The listing builds one solid part. Answer for the finished solid, in the listing's coordinates (mm). Face numbers are marked on the shaded views. Coordinates: 2 decimals unless noted, no trailing zeros. Order: outer loops, then holes, each group sorted by start corner. A loop starts at its lowest first (then second) coordinate and runs counter-clockwise, first axis right, second up. Notation, with made-up numbers: M 46.25,74.25 L 82.25,74.25 A8 cw 82.25,79.25 Z; hole C -21,-28.75 d1. An arc over 180 degrees is marked long. One line per item, written item: value. Start each with the question number.
Q1. Each of these flat-tipped pins is pushed along its axis until it touches: pin 1 Ø2 at (y, z) = (-5.5, -104) entering from -X; pin 2 Ø2 at (x, z) = (66.5, -6.5) entering from -Y; pin 3 Ø4 at (y, z) = (-22.5, -83) entering from -X. Where does it stop, or does it pass through?
Q2. Straight lines are drawn through the part: line 1 along X through (y, z) = (-5, -84); line 2 along Y through (x, z) = (62.5, -21.5); line 3 along Y through (x, z) = (81, -77). For each, find the intervals that lie inside material, in ascending order. Write a range as [from, to].
Q3. The part is cut by section A-A on y = -2. Give the vertices of the cut face in (x, z), then the cut area to 3 significant figures.
Q4. Determine the mould class of the marked faces 1 and 2 for opening direction Z: pulls with the +Z half, pulls with the -Z half, needs draft (parallel to the pull), parting line crosses it, or undercut.
```python
from build123d import *

# Parameters (mm, degrees)
SKETCH1_W                       = 24.199471414
SKETCH1_H                       = 2
BOSS_EXTRUDE1_DEPTH             = 35
BOSS_EXTRUDE1_DIRECTION_2_REACH = 26.277


with BuildPart() as part:
    # Sketch6 → Revolve3 (revolve)
    with BuildSketch(Plane.XY.offset(-46.235660898)):
        with BuildLine():
            Line((16.206828031, 19.733449427), (16.206828031, 24.27673627))
            add(Edge.make_bspline(
                [(100.543718281, 0), (66.637702737, 19.683925925), (36.295673337, 23.877083975), (16.206828031, 24.27673627)],
                knots=[0, 0, 0, 0, 1, 1, 1, 1], degree=3))
            add(Edge.make_bspline(
                [(16.206828031, 19.733449427), (44.550281864, 20.046720972), (71.658331759, 8.477286849), (100.543718281, 0)],
                knots=[0, 0, 0, 0, 1, 1, 1, 1], degree=3))
        make_face()
    revolve(axis=Axis((16.206828031, 19.733449427, -46.235660898), (0, 1, 0)))

    # Sketch1 → Boss-Extrude1 (add)
    with BuildSketch(Plane(origin=(0, 0, 0), x_dir=(1, 0, 0), z_dir=(0, 1, 0))):
        with Locations((19.440545507, 104.374561644)):
            Rectangle(SKETCH1_W, SKETCH1_H)
        Polygon((68.633841253, 77.067834217), (57.432693736, 91.113628939), (55.869030771, 89.866649335), (69.659558116, 72.573875009), align=None)
        Polygon((72.129937387, 19.465930814), (77.514826367, 43.058670955), (75.564970543, 43.503712823), (70.180081563, 19.910972681), align=None)
        Polygon((30.661981859, -13.103705945), (52.464952222, -2.603948803), (51.597184744, -0.802011068), (29.79421438, -11.301768209), align=None)
        Polygon((-20.656832908, -0.989589169), (1.146137456, -11.48934631), (2.013904934, -9.687408574), (-19.78906543, 0.812348567), align=None)
        Polygon((-43.18239268, 46.686104127), (-37.7975037, 23.093363986), (-35.847647875, 23.538405854), (-41.232536856, 47.131145995), align=None)
        Polygon((-19.952491512, 94.022604484), (-35.040615149, 75.102695874), (-33.476952184, 73.85571627), (-18.388828547, 92.77562488), align=None)
    extrude(amount=-BOSS_EXTRUDE1_DEPTH)

    # Sketch1 → Boss-Extrude1 direction 2 (add, up to next)
    with BuildSketch(Plane(origin=(0, 0, 0), x_dir=(1, 0, 0), z_dir=(0, 1, 0)), mode=Mode.PRIVATE) as boss_extrude1_direction_2_sk1:
        with Locations((19.440545507, 104.374561644)):
            Rectangle(SKETCH1_W, SKETCH1_H)
    boss_extrude1_direction_2_tool1 = extrude(boss_extrude1_direction_2_sk1.sketch, amount=BOSS_EXTRUDE1_DIRECTION_2_REACH, mode=Mode.PRIVATE) - part.part
    add(boss_extrude1_direction_2_tool1.solids().sort_by_distance((19.440546, 0, -104.374562))[0])
    # Sketch1 → Boss-Extrude1 direction 2 (add, up to next)
    with BuildSketch(Plane(origin=(0, 0, 0), x_dir=(1, 0, 0), z_dir=(0, 1, 0)), mode=Mode.PRIVATE) as boss_extrude1_direction_2_sk2:
        Polygon((68.633841253, 77.067834217), (57.432693736, 91.113628939), (55.869030771, 89.866649335), (69.659558116, 72.573875009), align=None)
    boss_extrude1_direction_2_tool2 = extrude(boss_extrude1_direction_2_sk2.sketch, amount=BOSS_EXTRUDE1_DIRECTION_2_REACH, mode=Mode.PRIVATE) - part.part
    add(boss_extrude1_direction_2_tool2.solids().sort_by_distance((62.894136, 0, -82.605929))[0])
    # Sketch1 → Boss-Extrude1 direction 2 (add, up to next)
    with BuildSketch(Plane(origin=(0, 0, 0), x_dir=(1, 0, 0), z_dir=(0, 1, 0)), mode=Mode.PRIVATE) as boss_extrude1_direction_2_sk3:
        Polygon((72.129937387, 19.465930814), (77.514826367, 43.058670955), (75.564970543, 43.503712823), (70.180081563, 19.910972681), align=None)
    boss_extrude1_direction_2_tool3 = extrude(boss_extrude1_direction_2_sk3.sketch, amount=BOSS_EXTRUDE1_DIRECTION_2_REACH, mode=Mode.PRIVATE) - part.part
    add(boss_extrude1_direction_2_tool3.solids().sort_by_distance((73.847454, 0, -31.484822))[0])
    # Sketch1 → Boss-Extrude1 direction 2 (add, up to next)
    with BuildSketch(Plane(origin=(0, 0, 0), x_dir=(1, 0, 0), z_dir=(0, 1, 0)), mode=Mode.PRIVATE) as boss_extrude1_direction_2_sk4:
        Polygon((30.661981859, -13.103705945), (52.464952222, -2.603948803), (51.597184744, -0.802011068), (29.79421438, -11.301768209), align=None)
    boss_extrude1_direction_2_tool4 = extrude(boss_extrude1_direction_2_sk4.sketch, amount=BOSS_EXTRUDE1_DIRECTION_2_REACH, mode=Mode.PRIVATE) - part.part
    add(boss_extrude1_direction_2_tool4.solids().sort_by_distance((41.129583, 0, 6.952859))[0])
    # Sketch1 → Boss-Extrude1 direction 2 (add, up to next)
    with BuildSketch(Plane(origin=(0, 0, 0), x_dir=(1, 0, 0), z_dir=(0, 1, 0)), mode=Mode.PRIVATE) as boss_extrude1_direction_2_sk5:
        Polygon((-20.656832908, -0.989589169), (1.146137456, -11.48934631), (2.013904934, -9.687408574), (-19.78906543, 0.812348567), align=None)
    boss_extrude1_direction_2_tool5 = extrude(boss_extrude1_direction_2_sk5.sketch, amount=BOSS_EXTRUDE1_DIRECTION_2_REACH, mode=Mode.PRIVATE) - part.part
    add(boss_extrude1_direction_2_tool5.solids().sort_by_distance((-9.321464, 0, 5.338499))[0])
    # Sketch1 → Boss-Extrude1 direction 2 (add, up to next)
    with BuildSketch(Plane(origin=(0, 0, 0), x_dir=(1, 0, 0), z_dir=(0, 1, 0)), mode=Mode.PRIVATE) as boss_extrude1_direction_2_sk6:
        Polygon((-43.18239268, 46.686104127), (-37.7975037, 23.093363986), (-35.847647875, 23.538405854), (-41.232536856, 47.131145995), align=None)
    boss_extrude1_direction_2_tool6 = extrude(boss_extrude1_direction_2_sk6.sketch, amount=BOSS_EXTRUDE1_DIRECTION_2_REACH, mode=Mode.PRIVATE) - part.part
    add(boss_extrude1_direction_2_tool6.solids().sort_by_distance((-39.51502, 0, -35.112255))[0])
    # Sketch1 → Boss-Extrude1 direction 2 (add, up to next)
    with BuildSketch(Plane(origin=(0, 0, 0), x_dir=(1, 0, 0), z_dir=(0, 1, 0)), mode=Mode.PRIVATE) as boss_extrude1_direction_2_sk7:
        Polygon((-19.952491512, 94.022604484), (-35.040615149, 75.102695874), (-33.476952184, 73.85571627), (-18.388828547, 92.77562488), align=None)
    boss_extrude1_direction_2_tool7 = extrude(boss_extrude1_direction_2_sk7.sketch, amount=BOSS_EXTRUDE1_DIRECTION_2_REACH, mode=Mode.PRIVATE) - part.part
    add(boss_extrude1_direction_2_tool7.solids().sort_by_distance((-26.714722, 0, -83.93916))[0])


solid = part.part
```
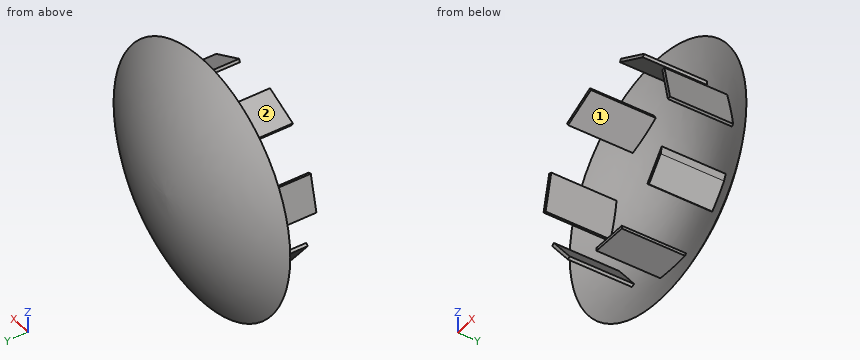
Output:
1. pin 1: stops at x = 7.34
1. pin 2: stops at y = 6.01
1. pin 3: stops at x = -30.34
2. line 1: x = [-27.95, -25.39], [60.55, 63.11]
2. line 2: y = [10.03, 14.74]
2. line 3: y = [3.88, 6.72]
3. outline: M -43.18,-46.69 L -41.23,-47.13 L -35.85,-23.54 L -37.8,-23.09 Z; M -35.04,-75.1 L -19.95,-94.02 L -18.39,-92.78 L -33.48,-73.86 Z; M -20.66,0.99 L -19.79,-0.81 L 2.01,9.69 L 1.15,11.49 Z; M 7.34,-105.37 L 31.54,-105.37 L 31.54,-103.37 L 7.34,-103.37 Z; M 29.79,11.3 L 51.6,0.8 L 52.46,2.6 L 30.66,13.1 Z; M 55.87,-89.87 L 57.43,-91.11 L 68.63,-77.07 L 69.66,-72.57 Z; M 70.18,-19.91 L 75.56,-43.5 L 77.51,-43.06 L 72.13,-19.47 Z
3. area: 330 mm^2
4. face 1: undercut
4. face 2: undercut
